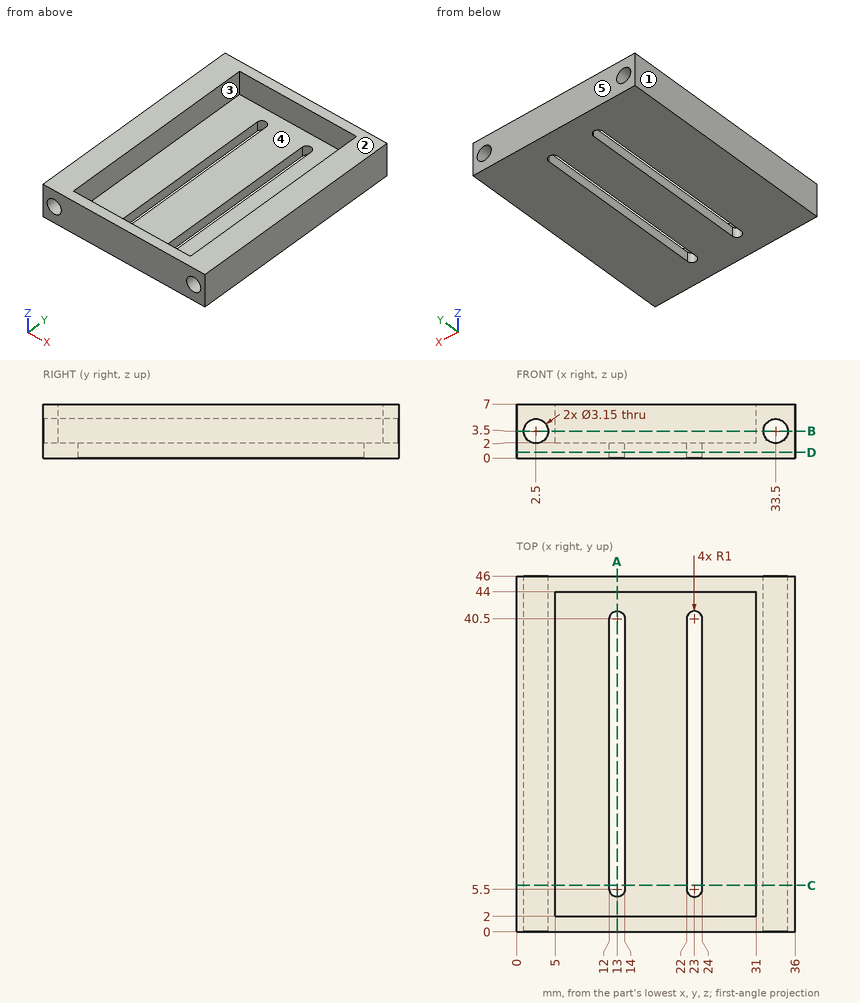
Can you work these out from the drawing? Everything is in mm from the part's minimum corner. A direction names the side the tool comes from. Give positions to 0.01 mm unless a question says otherwise; leave off trailing zeros. Loops run counter-clockwise (first coordinate to the right, second up) from the corner with the lowest first, then second, coordinate; pieces in that order, holes last. Notation, with made-up numbers: (32.5, 51) -> (54.5, 51) arc R16 cw to (54.5, 56) -> close; hole circle Ø2 at (63.5, 50). An arc over 180 degrees is marked (long way). Return JSON: item names as keys, results as strings.
Item 1: We'd pull the mould along X, two halves only. Please class the marked faces 1, 2 and 3: +X half, -X half, draft (parallel to the pull), parting line (faces both ways), or undercut.
Geometry results:
{"face 1": "-X half", "face 2": "draft", "face 3": "undercut"}
Item 2: If we section it at C-C on y = 6: List the corners of the cut face in (x, z) for me (3 decimals), plus the area to 3 significant figures.
Geometry results:
{"outline": "(0, 0) -> (12, 0) -> (12, 2) -> (5, 2) -> (5, 7) -> (0, 7) -> close; (14, 0) -> (22, 0) -> (22, 2) -> (14, 2) -> close; (24, 0) -> (36, 0) -> (36, 7) -> (31, 7) -> (31, 2) -> (24, 2) -> close; hole circle Ø3.15 at (2.5, 3.5); hole circle Ø3.15 at (33.5, 3.5)", "area": "98.4 mm²"}
Item 3: If we section it at A-A on x = 13: List the corners of the cut face in (y, z) for me, plus the area to 3 significant figures.
Geometry results:
{"outline": "(0, 0) -> (4.5, 0) -> (4.5, 2) -> (2, 2) -> (2, 7) -> (0, 7) -> close; (41.5, 0) -> (46, 0) -> (46, 7) -> (44, 7) -> (44, 2) -> (41.5, 2) -> close", "area": "38.0 mm²"}
Item 4: If we section it at B-B on z = 3.5: List the corners of the cut face in (x, y) for me (3 decimals).
Geometry results:
{"outline": "(0, 0) -> (0.925, 0) -> (0.925, 46) -> (0, 46) -> close; (4.075, 0) -> (31.925, 0) -> (31.925, 46) -> (4.075, 46) -> close; (35.075, 0) -> (36, 0) -> (36, 46) -> (35.075, 46) -> close; hole (5, 2) -> (31, 2) -> (31, 44) -> (5, 44) -> close"}
Item 5: Which directions (+Z, -Z, +X, -X, +Y, -Y) give clear straight access to the entire face, cutting with the end or side of a thin tool? Please do the marked faces 4 and 5.
Geometry results:
{"face 4": "+Z", "face 5": "+Z, -Z, +X, -X, +Y"}
Item 6: If we section it at D-D on z = 0.75: List the corners of the cut face in (x, y) for me.
Geometry results:
{"outline": "(0, 0) -> (36, 0) -> (36, 46) -> (0, 46) -> close; hole (12, 5.5) arc R1 ccw to (14, 5.5) -> (14, 40.5) arc R1 ccw to (12, 40.5) -> close; hole (22, 5.5) arc R1 ccw to (24, 5.5) -> (24, 40.5) arc R1 ccw to (22, 40.5) -> close"}
Item 7: I need wall thicknesses on L1, parallel to X at y = 10, z = 3.5 (3 decimals); L2, parallel to Y at x = 6, z = 4; L3, parallel to Z at x = 33.5, y = 33.5 (3 decimals). Which ranges of each line are inside material? Lowest first, please. Write a range as from..to.
Geometry results:
{"L1": "x = 0..0.925, 4.075..5, 31..31.925, 35.075..36", "L2": "y = 0..2, 44..46", "L3": "z = 0..1.925, 5.075..7"}
Item 8: I'm going to push a flat-ended pin straight in: pin 1 (1.5 mm diameter, centred on x = 12.5, y = 8.5, fed in from +Z). Where does the tip first touch, or does it pass through?
Geometry results:
{"pin 1": "stops at z = 2"}
